For this review, take the finished solid that the model builds, in its own axes (mm). Face numbers are marked on the shaded views. A direction names the side the tool comes from. Round coordinates to 2 decimals unless told otherwise and drop trailing zeros. Loops run counter-clockwise (first coordinate to the right, second up) from the corner with the lowest first, then second, coordinate; pieces in that order, holes last.
1) Take a section at A-A (x = -6). State the section outline as (y, z) points.
2) Tool access review of the marked faces 1, 2, 3 and 4: name each direction out of +Z, -Z, +X, -X, +Y, -Y from which nothing blocks a thin tool from reaching the whole face with its end or side.
3) Take a section at B-B (z = -49). State the section outline as (x, y) points, then the cut area to 3 significant figures.
4) Insertion check: pin 1 (8 mm diameter, centred on y = -38.5, z = -55, fed in from +X); pin 2 (8 mm diameter, centred on y = -34.5, z = -54, fed in from -X); pin 3 (4 mm diameter, centred on x = 28, y = -5.5, fed in from +Z); pin 4 (3.5 mm diameter, centred on y = -36.5, z = -40, fed in from +X). Each pin has a flat end and moves straight along its axis. Give the tip position at first contact, or say it passes through.
5) Take a section at C-C (x = 30.5). State the section outline as (y, z) points.
6) Wall thickness on L1, parallel to Z at x = -33, y = -45.5; L2, parallel to Y at x = -34, z = -38; L3, parallel to Z at x = -4, y = 15.5: over which ranges is each line inside the solid? List them lowest first.
7) Take a section at D-D (y = 20). State the section outline as (x, z) points, then the cut area to 3 significant figures.
8) Mouldability with a two-part tool opening along Z and no side actions: class the marked faces 5, 6, 7 and 8 as pulls with the +Z half, pulls with the -Z half, needs draft (parallel to the pull), parting line crosses it, or undercut.
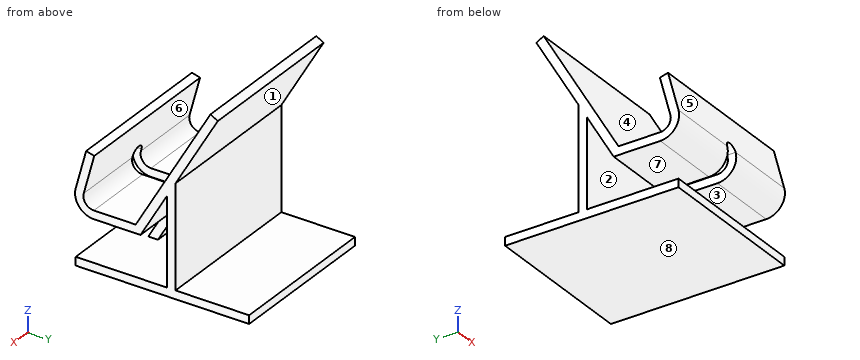
```python
from build123d import *

# Parameters (mm, degrees)
F1_DEPTH      = 37.5
F2_W          = 29.5
F2_H          = 20
F2_W_2        = 6
F2_H_2        = 11.3293714059
F3_DEPTH      = 43.7455051422
F3_DEPTH_BACK = 2


with BuildPart() as f1:
    # F0 (on Right) → F1 (new body, symmetric)
    with BuildSketch(Plane.YZ):
        with BuildLine():
            ThreePointArc((-49.1559958296, -42.4996678599), (-53.122762531, -40.5434750049), (-53.985624961, -36.2055726343))
            Line((-53.985624961, -36.2055726343), (-48.9735712256, -17.5003334434))
            Line((-48.9735712256, -17.5003334434), (-52.8372736915, -16.4650574879))
            Line((-52.8372736915, -16.4650574879), (-57.8493273667, -35.1702964539))
            ThreePointArc((-57.8493273667, -35.1702964539), (-56.2961749927, -42.9785207209), (-49.1559949301, -46.4996678599))
            Line((-49.1559949301, -46.4996678599), (-31.4653969064, -46.4996678599))
            Line((-31.4653969064, -46.4996678599), (-43.0124022901, -66.4996678599))
            Line((-43.0124022901, -66.4996678599), (-57.8493273667, -66.4996678599))
            Line((-57.8493273667, -66.4996678599), (-57.8493273667, -70.499666991))
            Line((-57.8493273667, -70.499666991), (25.1038222245, -70.499666991))
            Line((25.1038222245, -70.499666991), (25.1038222245, -66.4996678599))
            Line((25.1038222245, -66.4996678599), (-10.1038222245, -66.4996678599))
            Line((-10.1038222245, -66.4996678599), (-10.1038222245, -17.5003334434))
            Line((-10.1038222245, -17.5003334434), (10.1038222245, 17.5003334434))
            Line((10.1038222245, 17.5003334434), (6.6397213618, 19.500333009))
            Line((6.6397213618, 19.500333009), (-29.1559958296, -42.4996678599))
            Line((-29.1559958296, -42.4996678599), (-49.1559958296, -42.4996678599))
        make_face()
        Polygon((-14.1038222245, -66.4996678599), (-38.3936011399, -66.4996678599), (-14.1038222245, -24.4285366737), align=None, mode=Mode.SUBTRACT)
    extrude(amount=F1_DEPTH, both=True)

    # F2 (on face) → F3 (cut, two sides)
    with BuildSketch(Plane.XZ.offset(57.8493273667)) as f3_sk:
        with Locations((-22.75, -56.4996678599)):
            Rectangle(F2_W, F2_H)
        with Locations((22.75, -56.4996678599)):
            Rectangle(F2_W, F2_H)
        with Locations((0, -40.8349821569)):
            Rectangle(F2_W_2, F2_H_2)
        with BuildLine():
            Line((-3, -35.1702964539), (3, -35.1702964539))
            ThreePointArc((3, -35.1702964539), (0, -32.1702964539), (-3, -35.1702964539))
        make_face()
    extrude(amount=-F3_DEPTH, mode=Mode.SUBTRACT)
    extrude(f3_sk.sketch, amount=F3_DEPTH_BACK, mode=Mode.SUBTRACT)


solid = f1.part
```
Response:
1. outline: (-57.85, -70.5) - (25.1, -70.5) - (25.1, -66.5) - (-10.1, -66.5) - (-10.1, -17.5) - (10.1, 17.5) - (6.64, 19.5) - (-29.16, -42.5) - (-49.16, -42.5) arc R5 cw to (-53.99, -36.21) - (-48.97, -17.5) - (-52.84, -16.47) - (-57.85, -35.17) arc R9 ccw to (-49.16, -46.5) - (-31.47, -46.5) - (-43.01, -66.5) - (-57.85, -66.5) - close; hole (-38.39, -66.5) - (-14.1, -66.5) - (-14.1, -24.43) - close
2. face 1: +X, -X, +Y
2. face 2: +X, -X
2. face 3: +X, -Y
2. face 4: +Z, +X, -X
3. outline: (-37.5, -14.1) - (37.5, -14.1) - (37.5, -10.1) - (-37.5, -10.1) - close; (-8, -32.91) - (8, -32.91) - (8, -28.29) - (-8, -28.29) - close
3. area: 374 mm2
4. pin 1: stops at x = 8
4. pin 2: stops at x = -8
4. pin 3: stops at z = 1.94
4. pin 4: passes through
5. outline: (-57.85, -70.5) - (25.1, -70.5) - (25.1, -66.5) - (-10.1, -66.5) - (-10.1, -17.5) - (10.1, 17.5) - (6.64, 19.5) - (-29.16, -42.5) - (-49.16, -42.5) arc R5 cw to (-53.99, -36.21) - (-48.97, -17.5) - (-52.84, -16.47) - (-57.85, -35.17) arc R9 ccw to (-49.16, -46.5) - (-26.85, -46.5) - (-14.1, -24.43) - (-14.1, -66.5) - (-57.85, -66.5) - close
6. L1: z = -70.5 to -66.5, -46.5 to -42.5
6. L2: y = -58.14 to -54.13, -26.56 to -21.94, -14.1 to -10.1
6. L3: z = -70.5 to -66.5
7. outline: (-37.5, -70.5) - (37.5, -70.5) - (37.5, -66.5) - (-37.5, -66.5) - close
7. area: 300 mm2
8. face 5: pulls with the +Z half
8. face 6: undercut
8. face 7: undercut
8. face 8: pulls with the -Z half
